from build123d import *

# Parameters (mm, degrees)
SKETCH1_W           = 20
SKETCH1_H           = 17.5
BOSS_EXTRUDE1_DEPTH = 1.3
FILLET1_R           = 3
CUT_EXTRUDE1_DEPTH  = 26.902339963
SKETCH2_3_W         = 1.4
SKETCH2_3_H         = 10
BOSS_EXTRUDE2_DEPTH = 1.3
SKETCH3_W           = 20
SKETCH3_H           = 2
CUT_EXTRUDE2_DEPTH  = 26.902339963
CUT_EXTRUDE3_DEPTH  = 26.902339963


with BuildPart() as part:
    # Sketch1 → Boss-Extrude1 (new body)
    with BuildSketch(Plane.XY):
        Rectangle(SKETCH1_W, SKETCH1_H)
        Polygon((-15.556349186, 14.306349186), (-10, 8.75), (10, 8.75), (15.556349186, 14.306349186), (7.071067812, 22.79163056), (0, 15.720562748), (-7.071067812, 22.79163056), align=None)
    extrude(amount=BOSS_EXTRUDE1_DEPTH)

    # Fillet1
    fillet1_edges = [part.edges().sort_by_distance(p)[0] for p in [
        (10, 8.75, 0.65),
        (-10, 8.75, 0.65),
        (-15.556349186, 14.306349186, 0.65),
        (-7.071067812, 22.79163056, 0.65),
        (7.071067812, 22.79163056, 0.65),
        (15.556349186, 14.306349186, 0.65),
    ]]
    fillet(fillet1_edges, radius=FILLET1_R)

    # Sketch2 → Cut-Extrude1 (cut, through all)
    with BuildSketch(Plane.XY.offset(1.3)):
        Polygon((7.071067812, 19.963203436), (12.727922061, 14.306349186), (12.02081528, 13.599242405), (6.363961031, 19.256096654), align=None)
        Polygon((-12.727922061, 14.306349186), (-12.02081528, 13.599242405), (-6.363961031, 19.256096654), (-7.071067812, 19.963203436), align=None)
    extrude(amount=-CUT_EXTRUDE1_DEPTH, mode=Mode.SUBTRACT)

    # Sketch2_3 → Boss-Extrude2 (add)
    with BuildSketch(Plane.XY.offset(1.3)):
        with Locations((-10.7, 0)):
            Rectangle(SKETCH2_3_W, SKETCH2_3_H)
        with Locations((10.7, 0)):
            Rectangle(SKETCH2_3_W, SKETCH2_3_H)
    extrude(amount=-BOSS_EXTRUDE2_DEPTH)

    # Sketch3 → Cut-Extrude2 (cut, through all)
    with BuildSketch(Plane.XY.offset(1.3)):
        with Locations((0, -7.75)):
            Rectangle(SKETCH3_W, SKETCH3_H)
    extrude(amount=-CUT_EXTRUDE2_DEPTH, mode=Mode.SUBTRACT)

    # Sketch4 → Cut-Extrude3 (cut, through all)
    with BuildSketch(Plane.XY.offset(1.3)):
        Polygon((-4.949747468, 17.841883092), (-0.707106781, 13.599242405), (-1.414213562, 12.892135624), (-5.656854249, 17.134776311), align=None)
        Polygon((1.414213562, 12.892135624), (5.656854249, 17.134776311), (4.949747468, 17.841883092), (0.707106781, 13.599242405), align=None)
    extrude(amount=-CUT_EXTRUDE3_DEPTH, mode=Mode.SUBTRACT)


solid = part.part
The model under review builds one solid part; all positions refer to its coordinate system, in mm. A direction names the side the tool comes from. Round coordinates to 2 decimals unless told otherwise and drop trailing zeros. Write each loop counter-clockwise with the first axis right and the second up, starting at its lowest first coordinate (ties: lowest second). Pieces come first, ordered by that corner, then holes. Notation, with made-up numbers: (-11, -34.75) -> (8, -34.75) arc R26 ccw to (8, -20.75) -> close; hole circle Ø1 at (-11, 3.25). An arc over 180 degrees is marked (long way). Answer as a JSON object with one key per item and string values.
1. Machinability: for faces 1 (the face through (-2.44, 18.16, 0.64)), 2 (the face through (-10, 6, 1)), 3 (the face through (-9.86, 17.174, 0.659)), which of the approach directions +Z, -Z, +X, -X, +Y, -Y give a long, thin tool a straight path to every point of the face, cutting with its end or side? Answer none if there is none.
Results found:
{"face 1": "+Z, -Z, +Y", "face 2": "+Z, -Z, -X", "face 3": "+Z, -Z"}
2. The part is to be moulded in two halves that separate along X. For faces 4 (the face through (10, -6, 1)), 5 (the face through (7.1, 21.55, 0.66)), 6 (the face through (-11.28, 18.58, 0.64)), say which applies: pulls with the +X half, pulls with the -X half, needs draft (parallel to the pull), parting line crosses it, or undercut.
Results found:
{"face 4": "pulls with the +X half", "face 5": "undercut", "face 6": "pulls with the -X half"}
3. We need section C-C on x = -3.75. State the section outline as (y, z) points.
Results found:
{"outline": "(-6.75, 0) -> (15.23, 0) -> (15.23, 1.3) -> (-6.75, 1.3) -> close; (16.64, 0) -> (19.47, 0) -> (19.47, 1.3) -> (16.64, 1.3) -> close"}
4. To check wall thickness, follow line 1 along X through (y, z) = (2, 0.95); line 2 along Y through (x, z) = (3.5, 0.35); line 3 along Y through (x, z) = (-5, 0.4). State the ranges of each line that lie inside material, in increasing order.
Results found:
{"line 1": "x = -11.4 to 11.4", "line 2": "y = -6.75 to 14.98, 16.39 to 19.22", "line 3": "y = -6.75 to 16.48, 17.79 to 20.72"}
5. Clearance check with flat-ended pins moving along their axes: pin 1 (0.6 mm diameter, centred on y = 6, z = 1, fed in from +X); pin 2 (0.6 mm diameter, centred on y = 2, z = 0.5, fed in from +X). State where each tip first meets the part, or that it passes through.
Results found:
{"pin 1": "stops at x = 10", "pin 2": "stops at x = 11.4"}
6. We need section A-A on y = 15. State the section outline as (x, z) points, and give its area (3 significant figures).
Results found:
{"outline": "(-14.23, 0) -> (-12.03, 0) -> (-12.03, 1.3) -> (-14.23, 1.3) -> close; (-10.62, 0) -> (-3.52, 0) -> (-3.52, 1.3) -> (-10.62, 1.3) -> close; (-2.11, 0) -> (2.11, 0) -> (2.11, 1.3) -> (-2.11, 1.3) -> close; (3.52, 0) -> (10.62, 0) -> (10.62, 1.3) -> (3.52, 1.3) -> close; (12.03, 0) -> (14.23, 0) -> (14.23, 1.3) -> (12.03, 1.3) -> close", "area": "29.7 mm^2"}
7. We need section D-D on z = 0.75. State how many separate pieces and enclosed holes the cut face has, and give its area (3 significant figures).
Results found:
{"separate pieces": "1", "enclosed holes": "4", "area": "587 mm^2"}
8. We need section B-B on x = -10.5. State the section outline as (y, z) points.
Results found:
{"outline": "(-5, 0) -> (5, 0) -> (5, 1.3) -> (-5, 1.3) -> close; (9.17, 0) -> (15.12, 0) -> (15.12, 1.3) -> (9.17, 1.3) -> close; (16.53, 0) -> (19.36, 0) -> (19.36, 1.3) -> (16.53, 1.3) -> close"}
